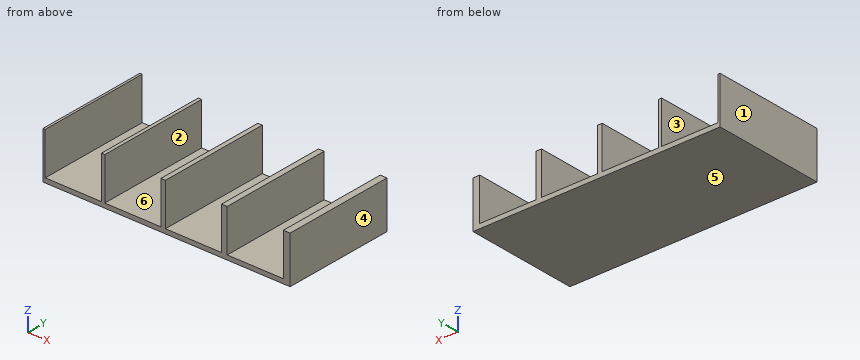
```python
from build123d import *

# Parameters (mm, degrees)
F0_W     = 88
F0_H     = 40
F1_DEPTH = 1.6
F2_W     = 0.8
F2_H     = 40
F2_W_2   = 1.2
F2_W_3   = 1.6
F2_W_4   = 2
F2_W_5   = 2.4
F3_DEPTH = 15


with BuildPart() as f1:
    # F0 (on Top) → F1 (new body)
    with BuildSketch(Plane.XY):
        with Locations((44, -20)):
            Rectangle(F0_W, F0_H)
    extrude(amount=F1_DEPTH)

    # F2 (on face) → F3 (join)
    with BuildSketch(Plane.XY.offset(1.6)):
        with Locations((0.4, -20)):
            Rectangle(F2_W, F2_H)
        with Locations((21.4, -20)):
            Rectangle(F2_W_2, F2_H)
        with Locations((42.8, -20)):
            Rectangle(F2_W_3, F2_H)
        with Locations((64.6, -20)):
            Rectangle(F2_W_4, F2_H)
        with Locations((86.8, -20)):
            Rectangle(F2_W_5, F2_H)
    extrude(amount=F3_DEPTH)


solid = f1.part
```
Work out the finished part from the listing and answer in its coordinate system (mm). Face numbers are marked on the shaded views. A direction names the side the tool comes from. Give positions to 0.01 mm unless a question says otherwise; leave off trailing zeros. Loops run counter-clockwise (first coordinate to the right, second up) from the corner with the lowest first, then second, coordinate; pieces in that order, holes last. Notation, with made-up numbers: (56, 7.25) - (68, 7.25) arc R28 cw to (68, 28.25) - close; hole circle Ø3 at (6, -6). An arc over 180 degrees is marked (long way). Use CSV: the item, a comma, the result in double quotes. Start each with the question number.
(1) A tool of negligible diameter and unlimited length cuts with its end or side. For the marked faces 5 and 6, from which of +Z, -Z, +X, -X, +Y, -Y can it reach the whole face along a straight path? Write none if from no direction.
(2) This flat-tipped pin is pushed along its axis until it touches: pin 1 (6 mm diameter, centred on x = 77.5, y = -26, fed in from +Z). Where does it stop, or does it pass through?
(3) Determine the mould class of the marked faces 1, 2, 3 and 4 for opening direction X: released by +X, released by -X, zero draft, split by the parting line, or undercut.
(4) Find section A-A, the plane z = 7.5. Determine the outline of the cut face in (x, y), plus the area to 3 significant figures.
(5) Find the intervals of material crossed by L1, parallel to X at y = -32, z = 6.25; L2, parallel to Z at x = 4.5, y = -35, in increasing order.
(6) Find section B-B, the plane y = -37. Determine the outline of the cut face in (x, z).
(7) Find section C-C, the plane x = 11. Determine the outline of the cut face in (y, z).
Results found:
1,face 5,"-Z, +X, -X, +Y, -Y"
1,face 6,"+Z, +Y, -Y"
2,pin 1,"z = 1.6"
3,face 1,"released by -X"
3,face 2,"undercut"
3,face 3,"undercut"
3,face 4,"released by +X"
4,outline,"(0, -40) - (0.8, -40) - (0.8, 0) - (0, 0) - close; (20.8, -40) - (22, -40) - (22, 0) - (20.8, 0) - close; (42, -40) - (43.6, -40) - (43.6, 0) - (42, 0) - close; (63.6, -40) - (65.6, -40) - (65.6, 0) - (63.6, 0) - close; (85.6, -40) - (88, -40) - (88, 0) - (85.6, 0) - close"
4,area,"320 mm^2"
5,L1,"0 to 0.8, 20.8 to 22, 42 to 43.6, 63.6 to 65.6, 85.6 to 88"
5,L2,"0 to 1.6"
6,outline,"(0, 0) - (88, 0) - (88, 16.6) - (85.6, 16.6) - (85.6, 1.6) - (65.6, 1.6) - (65.6, 16.6) - (63.6, 16.6) - (63.6, 1.6) - (43.6, 1.6) - (43.6, 16.6) - (42, 16.6) - (42, 1.6) - (22, 1.6) - (22, 16.6) - (20.8, 16.6) - (20.8, 1.6) - (0.8, 1.6) - (0.8, 16.6) - (0, 16.6) - close"
7,outline,"(-40, 0) - (0, 0) - (0, 1.6) - (-40, 1.6) - close"
